Check sheet for the modelled part. Datum: model origin and axes. Units: mm. A direction names the side the tool comes from. Round coordinates to 2 decimals unless told otherwise and drop trailing zeros. Write each loop counter-clockwise with the first axis right and the second up, starting at its lowest first coordinate (ties: lowest second). Pieces come first, ordered by that corner, then holes. Notation, with made-up numbers: (-7, 72.25) - (47, 72.25) arc R15 cw to (47, 76.25) - close; hole circle Ø2 at (5, 6). An arc over 180 degrees is marked (long way). Use one line per item in the form item = value. Start each with the question number.
1) Section check B-B (y = 166.5). Record the boundary of the cut face in (x, z) (1 decimal), then the cut area to 3 significant figures.
2) Scan lines: probe 1 along Z at (x, y) = (-10, 178) (1 decimal); probe 2 along X at (y, z) = (381, -78.9); probe 3 along X at (y, z) = (106, -30.5). Record each from-to range of solid material in increasing order.
3) Section check C-C (z = -16). Record the boundary of the cut face in (x, y).
4) Draft check along Z on faces 1 (the face through (-26, 200, 0)), 2 (the face through (-50.8, 200, -40)), 3 (the face through (-51, 0, -52)). Enter one of: +Z half, -Z half, draft (parallel to the pull), parting line (faces both ways), or undercut.
5) Gauge pin test, flat ends, axial feed: P1, Ø5, axis at x = -26.99, y = 25.4, coming from the +Z side; P2, Ø6, axis at y = 209, z = -11.5, coming from the +X side. Record the tip position at first contact, or that the pin passes through.
6) Section check A-A (x = -43). Record the boundary of the cut face in (y, z) (1 decimal).
7) Set-up check for faces 4 (the face through (-25, 200, -77.788)), 5 (the face through (-7.871, 8.273, -78.57)): record each of +Z, -Z, +X, -X, +Y, -Y from which the full face is reachable in a straight line by a thin tool's end or side.
8) Section check D-D (x = -19.5). Record the boundary of the cut face in (y, z) (1 decimal).
from build123d import *

# Parameters (mm, degrees)
BOSS_EXTRUDE1_DEPTH = 406.4
CUT_EXTRUDE1_DEPTH  = 406.4
SKETCH3_R           = 2.778125
CUT_EXTRUDE2_DEPTH  = 406.4


with BuildPart() as part:
    # Sketch1 → Boss-Extrude1 (new body)
    with BuildSketch(Plane(origin=(0, 0, 0), x_dir=(1, 0, 0), z_dir=(0, 1, 0))):
        Polygon((0, 0), (-52.3875, 0), (-52.3875, 79.375), (0, 79.375), (0, 77.7875), (-50.8, 77.7875), (-50.8, 1.5875), (0, 1.5875), align=None)
    extrude(amount=BOSS_EXTRUDE1_DEPTH)

    # Sketch2 → Cut-Extrude1 (cut)
    with BuildSketch(Plane.XY):
        with BuildLine():
            Line((0, 0), (0, 26.19375))
            ThreePointArc((0, 26.19375), (-8.070831371, 8.070831371), (-26.19375, 0))
            Line((-26.19375, 0), (0, 0))
        make_face()
        with BuildLine():
            Line((0, 382.011163771), (0, 406.4))
            Line((0, 406.4), (-24.388836229, 406.4))
            ThreePointArc((-24.388836229, 406.4), (-7.396266769, 399.003733231), (0, 382.011163771))
        make_face()
    extrude(amount=-CUT_EXTRUDE1_DEPTH, mode=Mode.SUBTRACT)

    # Sketch3 → Cut-Extrude2 (cut)
    with BuildSketch(Plane.XY):
        with Locations((-26.9875, 381)):
            Circle(SKETCH3_R)
        with Locations((-26.9875, 25.4)):
            Circle(SKETCH3_R)
    extrude(amount=-CUT_EXTRUDE2_DEPTH, mode=Mode.SUBTRACT)


solid = part.part
Results are:
q1.outline = (-52.4, -79.4) - (0, -79.4) - (0, -77.8) - (-50.8, -77.8) - (-50.8, -1.6) - (0, -1.6) - (0, 0) - (-52.4, 0) - close
q1.area = 287 mm²
q2.probe_1 = -79.4 to -77.8, -1.6 to 0
q2.probe_2 = -52.39 to -29.77, -24.21 to 0
q2.probe_3 = -52.39 to -50.8
q3.outline = (-52.39, 0) - (-50.8, 0) - (-50.8, 406.4) - (-52.39, 406.4) - close
q4.face_1 = +Z half
q4.face_2 = undercut
q4.face_3 = draft
q5.P1 = through
q5.P2 = -50.8
q6.outline = (0, -79.4) - (406.4, -79.4) - (406.4, -77.8) - (0, -77.8) - close; (0, -1.6) - (406.4, -1.6) - (406.4, 0) - (0, 0) - close
q7.face_4 = +X, +Y, -Y
q7.face_5 = +Z, -Z, +X, -Y
q8.outline = (1.2, -79.4) - (405.7, -79.4) - (405.7, -77.8) - (1.2, -77.8) - close; (1.2, -1.6) - (405.7, -1.6) - (405.7, 0) - (1.2, 0) - close
